Design review of the part built by this model. Coordinates are the model's own, in mm. A direction names the side the tool comes from. Round coordinates to 2 decimals unless told otherwise and drop trailing zeros. Loops run counter-clockwise (first coordinate to the right, second up) from the corner with the lowest first, then second, coordinate; pieces in that order, holes last. Notation, with made-up numbers: (-35.75, 72.25) -> (9.25, 72.25) arc R22 ccw to (9.25, 88.25) -> close; hole circle Ø4 at (54, 51). An arc over 180 degrees is marked (long way). Answer as CSV lines item,"result". Start each with the question number.
(1) For P1, Ø12.5, axis at x = -40, z = 7, coming from the -Y side; P2, Ø7.5, axis at y = 32, z = 6.5, coming from the +X side; P3, Ø8, axis at y = 21.5, z = 14.5, coming from the -X side, all flat-tipped, find the tip position at first contact; note any pin that passes through.
(2) Take a section at D-D, the plane x = -27. Write out the cut boundary in (y, z), and give its area (3 significant figures).
(3) Take a section at A-A, the plane x = 43. Write out the cut boundary in (y, z).
(4) Draft analysis for pull direction X (two halves, no side actions). For faces 1 (the face through (-15, -35, 10)), 2 (the face through (25, -10, 12)), 3 (the face through (-35, 25, 10)), 4 (the face through (-5, 35, 10)), state which applies: +X half, -X half, draft (parallel to the pull), parting line (faces both ways), or undercut.
(5) Machinability: for faces 5 (the face through (5, 35, 10)), 6 (the face through (-22, 0, 12)), 7 (the face through (-35, 5, 10)), which of the approach directions +Z, -Z, +X, -X, +Y, -Y give a long, thin tool a straight path to every point of the face, cutting with its end or side? Answer none if there is none.
(6) Take a section at B-B, the plane x = 1. Write out the cut boundary in (y, z).
(7) To check wall thickness, follow line 1 (X direction, y = 31.5, z = 5.5); line 2 (Z direction, x = -14, y = 6). State the ranges of each line that lie inside material, in increasing order. Write a range as from..to.
from build123d import *

# Parameters (mm, degrees)
F0_W      = 50
F0_H      = 50
F1_DEPTH  = 25
F2_T      = -3
F3_W      = 10
F3_H      = 25
F4_DEPTH  = 25
F6_DEPTH  = 50
F7_W      = 10
F7_H      = 25
F8_DEPTH  = 25
F10_DEPTH = 50
F11_W     = 10
F11_H     = 25
F12_DEPTH = 25
F14_DEPTH = 50
F15_W     = 10
F15_H     = 25
F16_DEPTH = 25
F18_DEPTH = 50


with BuildPart() as f1:
    # F0 (on Top) → F1 (new body)
    with BuildSketch(Plane.XY):
        Rectangle(F0_W, F0_H)
    extrude(amount=F1_DEPTH)

    # F2 (hollow: no face is removed)
    offset(amount=F2_T, mode=Mode.SUBTRACT)

    # F3 (on face) → F4 (join)
    with BuildSketch(Plane.YZ.offset(25)):
        with Locations((-20, 12.5)):
            Rectangle(F3_W, F3_H)
        with Locations((0, 12.5)):
            Rectangle(F3_W, F3_H)
        with Locations((20, 12.5)):
            Rectangle(F3_W, F3_H)
    extrude(amount=F4_DEPTH)

    # F5 (on face) → F6 (cut)
    with BuildSketch(Plane.XZ.offset(25)):
        Polygon((50, 0), (50, 25), (25, 25), align=None)
    extrude(amount=-F6_DEPTH, mode=Mode.SUBTRACT)

    # F7 (on face) → F8 (join)
    with BuildSketch(Plane(origin=(0, 25, 0), x_dir=(-1, 0, 0), z_dir=(0, 1, 0))):
        with Locations((-20, 12.5)):
            Rectangle(F7_W, F7_H)
        with Locations((0, 12.5)):
            Rectangle(F7_W, F7_H)
        with Locations((20, 12.5)):
            Rectangle(F7_W, F7_H)
    extrude(amount=F8_DEPTH)

    # F9 (on face) → F10 (cut)
    with BuildSketch(Plane(origin=(-25, 0, 0), x_dir=(0, -1, 0), z_dir=(-1, 0, 0))):
        Polygon((-25, 25), (-50, 25), (-50, 0), align=None)
    extrude(amount=-F10_DEPTH, mode=Mode.SUBTRACT)

    # F11 (on face) → F12 (join)
    with BuildSketch(Plane.XZ.offset(25)):
        with Locations((-20, 12.5)):
            Rectangle(F11_W, F11_H)
        with Locations((0, 12.5)):
            Rectangle(F11_W, F11_H)
        with Locations((20, 12.5)):
            Rectangle(F11_W, F11_H)
    extrude(amount=F12_DEPTH)

    # F13 (on face) → F14 (cut)
    with BuildSketch(Plane(origin=(-25, 0, 0), x_dir=(0, -1, 0), z_dir=(-1, 0, 0))):
        Polygon((50, 0), (50, 25), (25, 25), align=None)
    extrude(amount=-F14_DEPTH, mode=Mode.SUBTRACT)

    # F15 (on face) → F16 (join)
    with BuildSketch(Plane(origin=(-25, 0, 0), x_dir=(0, -1, 0), z_dir=(-1, 0, 0))):
        with Locations((-20, 12.5)):
            Rectangle(F15_W, F15_H)
        with Locations((0, 12.5)):
            Rectangle(F15_W, F15_H)
        with Locations((20, 12.5)):
            Rectangle(F15_W, F15_H)
    extrude(amount=F16_DEPTH)

    # F17 (on face) → F18 (cut)
    with BuildSketch(Plane(origin=(0, 25, 0), x_dir=(-1, 0, 0), z_dir=(0, 1, 0))):
        Polygon((50, 25), (25, 25), (50, 0), align=None)
    extrude(amount=-F18_DEPTH, mode=Mode.SUBTRACT)


solid = f1.part
The answers:
1,P1,"y = -25"
1,P2,"x = 25"
1,P3,"x = -39.5"
2,outline,"(-25, 0) -> (-15, 0) -> (-15, 23) -> (-25, 23) -> close; (-5, 0) -> (5, 0) -> (5, 23) -> (-5, 23) -> close; (15, 0) -> (25, 0) -> (25, 23) -> (15, 23) -> close"
2,area,"690 mm²"
3,outline,"(-25, 0) -> (-15, 0) -> (-15, 7) -> (-25, 7) -> close; (-5, 0) -> (5, 0) -> (5, 7) -> (-5, 7) -> close; (15, 0) -> (25, 0) -> (25, 7) -> (15, 7) -> close"
4,face 1,"undercut"
4,face 2,"+X half"
4,face 3,"draft"
4,face 4,"undercut"
5,face 5,"+Z, -Z, +Y"
5,face 6,"none"
5,face 7,"+Z, -Z, -X"
6,outline,"(-50, 0) -> (50, 0) -> (25, 25) -> (-25, 25) -> close; hole (-22, 3) -> (22, 3) -> (22, 22) -> (-22, 22) -> close"
7,line 1,"-25..-15, -5..5, 15..25"
7,line 2,"0..3, 22..25"
